Build history of the part. All positions in model axes, mm. Face numbers are marked on the shaded views. A direction names the side the tool comes from. Coordinates: 2 decimals unless noted, no trailing zeros. Order: outer loops, then holes, each group sorted by start corner. A loop starts at its lowest first (then second) coordinate and runs counter-clockwise, first axis right, second up. Notation, with made-up numbers: (4, 50) - (63, 50) arc R32 ccw to (63, 80) - close; hole circle Ø9 at (10, 43.5). An arc over 180 degrees is marked (long way). Write each question's results on one line, items separated by ' | '. Start each with the question number.
from build123d import *

# Parameters (mm, degrees)
EXTRUDE_1_DEPTH     = 8
SKETCH_2_R          = 1.5
EXTRUDE_2_DEPTH     = 10
M3X0_51_D           = 2.5
M3X0_51_DEPTH       = 6
M3X0_51_CSINK_D     = 3
M3X0_51_CSINK_ANGLE = 90
M3X0_51_TIP         = 0.751075774
CHAMFER_1_SIZE      = 0.5


with BuildPart() as part:
    # Эскиз1 → Вытянуть1 (new body)
    with BuildSketch(Plane.XY):
        Polygon((0, 4.041451884), (-3.5, 2.020725942), (-3.5, -2.020725942), (0, -4.041451884), (3.5, -2.020725942), (3.5, 2.020725942), align=None)
    extrude(amount=EXTRUDE_1_DEPTH)

    # Эскиз2 → Вытянуть2 (add)
    with BuildSketch(Plane.XY.offset(8)):
        Circle(SKETCH_2_R)
    extrude(amount=EXTRUDE_2_DEPTH)

    # Сверление под метчик M3x0.51
    with Locations(Plane(origin=(0, 0, 0), x_dir=(-1, 0, 0), z_dir=(0, 0, -1))):
        with Locations((0, 0)):
            CounterSinkHole(M3X0_51_D / 2, M3X0_51_CSINK_D / 2, depth=M3X0_51_DEPTH, counter_sink_angle=M3X0_51_CSINK_ANGLE)
            with Locations((0, 0, -(M3X0_51_DEPTH + M3X0_51_TIP / 2))):  # 118° drill point
                Cone(0, M3X0_51_D / 2, M3X0_51_TIP, mode=Mode.SUBTRACT)

    # Фаска1
    chamfer_1_edges = [part.edges().sort_by_distance(p)[0] for p in [
        (-1.5, 0, 18),
    ]]
    chamfer(chamfer_1_edges, length=CHAMFER_1_SIZE)


solid = part.part
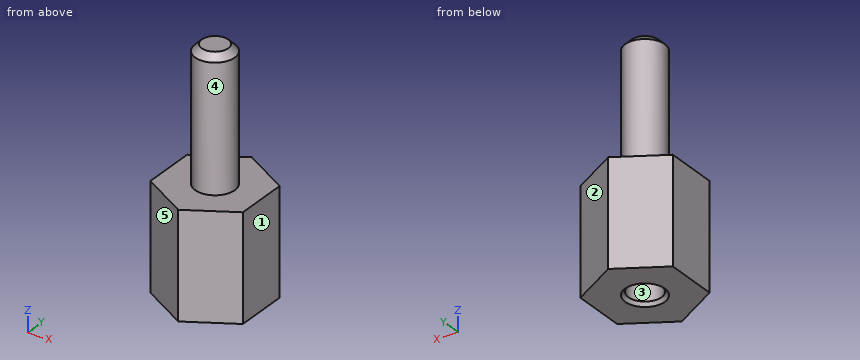
Item 1: Slice it at A-A (z = 4.25). Write the cut outline in (x, y), then the cut area to 3 significant figures.
Item 2: Slice it at D-D (x = 2.75). Write the cut outline in (y, z).
Item 3: Slice it at B-B (z = 16.75). Write the cut outline in (x, y).
Item 4: Pull direction Y, two halves, no side cores. Call the marked faces 1, 2 and 3: released by +Y, released by -Y, zero draft, split by the parting line, or undercut.
Item 5: Probe probe 1 along X at (y, z) = (0, 3.3); probe 2 along Z at (x, y) = (3, -0.75); probe 3 along Z at (x, y) = (-0.5, -1). List the from-to ranges inside material, lowest first.
Item 6: Which spindle directions (+Z, -Z, +X, -X, +Y, -Y) get a long thin tool onto all of the face, cutting with end or side? Do the marked faces 4 and 5. Say none if no direction does.
Item 7: Slice it at C-C (x = 2). Write the cut outline in (y, z).
Item 8: Flat gauge pins, fed straight in: P1, Ø4, axis at x = 1.5, z = 12.5, coming from the -Y side; P2, Ø2, axis at x = -2, z = 7, coming from the +Y side; P3, Ø2, axis at x = 2, y = -1, coming from the -Z side. Where does each tip first touch, or does it go through?
Resolved:
1) outline: (-3.5, -2.02) - (0, -4.04) - (3.5, -2.02) - (3.5, 2.02) - (0, 4.04) - (-3.5, 2.02) - close; hole circle Ø2.5 at (0, 0) | area: 37.5 mm^2
2) outline: (-2.45, 0) - (2.45, 0) - (2.45, 8) - (-2.45, 8) - close
3) outline: circle Ø3 at (0, 0)
4) face 1: zero draft | face 2: released by +Y | face 3: undercut
5) probe 1: -3.5 to -1.25, 1.25 to 3.5 | probe 2: 0 to 8 | probe 3: 6.08 to 17.88
6) face 4: +Z | face 5: +Z, -Z, -X, -Y
7) outline: (-2.89, 0) - (2.89, 0) - (2.89, 8) - (-2.89, 8) - close
8) P1: y = -1.5 | P2: y = 3.46 | P3: z = 0
